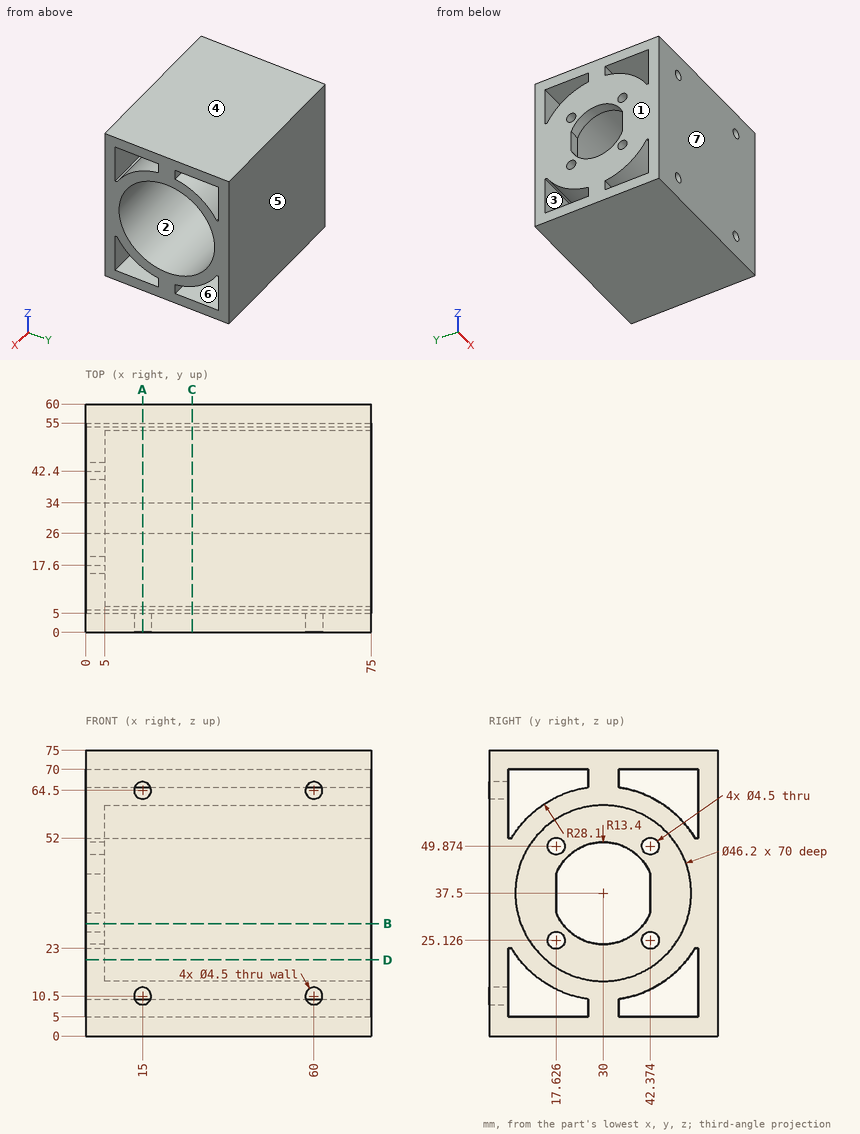
Answer from the drawing. Dimensions are ordinates in mm from the lowest x, y and z of the part. A direction names the side the tool comes from. Give positions to 0.01 mm unless a question says otherwise; leave off trailing zeros. Order: outer loops, then holes, each group sorted by start corner. A loop starts at its lowest first (then second) coordinate and runs counter-clockwise, first axis right, second up. Notation, with made-up numbers: (69, 73) - (78, 73) arc R11 cw to (78, 80) - close; hole circle Ø5 at (9.5, 60.25). An arc over 180 degrees is marked (long way). One line per item, written item: value. Start each with the question number.
1. Section C-C, the plane x = 28 is taken. Write down the section's boundary in (y, z), then the cut area to 3 significant figures.
2. Which of the six approach directions +Z, -Z, +X, -X, +Y, -Y give full straight-line access (tool end or side, diameter ignored) to the marked faces 1, 2 and 3?
3. Section A-A, the plane x = 15 is taken. Count the separate pieces of the cut face and the enclosed holes in it, then the cut area to 3 significant figures.
4. For a pull along Y with two mould halves and no side action, classify the marked faces 4, 5, 6 and 7 as released by +Y, released by -Y, zero draft, split by the parting line, or undercut.
5. Consider line 1 (X direction, y = 1.85, z = 10.5); line 2 (Y direction, x = 72.5, z = 57) (1 decimal); line 3 (Z direction, x = 69.5, y = 46.5) (1 decimal). Determine where each line is inside the solid, lowest interval first.
6. This flat-tipped pin is pushed along its axis until it touches: pin 1 Ø10 at (y, z) = (26, 34) entering from -X. Where does it stop, or does it pass through?
7. Section D-D, the plane z = 20 is taken. Write down the section's boundary in (x, y) (1 decimal).
8. Section B-B, the plane z = 29.5 is taken. Write down the section's boundary in (x, y).
Filled sheet:
1. outline: (0, 0) - (60, 0) - (60, 75) - (0, 75) - close; hole (5, 5) - (26, 5) - (26, 9.69) arc R28.1 cw to (5.93, 23) - (5, 23) - close; hole (5, 52) - (5.93, 52) arc R28.1 cw to (26, 65.31) - (26, 70) - (5, 70) - close; hole circle Ø46.2 at (30, 37.5); hole (34, 5) - (55, 5) - (55, 23) - (54.07, 23) arc R28.1 cw to (34, 9.69) - close; hole (34, 65.31) arc R28.1 cw to (54.07, 52) - (55, 52) - (55, 70) - (34, 70) - close
1. area: 2,020 mm²
2. face 1: +Z, -Z, -X, +Y, -Y
2. face 2: +X
2. face 3: +X, -X
3. separate pieces: 1
3. enclosed holes: 3
3. area: 1,980 mm²
4. face 4: zero draft
4. face 5: released by +Y
4. face 6: undercut
4. face 7: released by -Y
5. line 1: 0 to 12.75, 17.25 to 57.75, 62.25 to 75
5. line 2: 0 to 5, 9.8 to 17.6, 42.4 to 50.2, 55 to 60
5. line 3: 0 to 5, 14.8 to 21.3, 53.7 to 60.2, 70 to 75
6. pin 1: through
7. outline: (0, 0) - (75, 0) - (75, 5) - (0, 5) - close; (0, 8) - (75, 8) - (75, 14.9) - (5, 14.9) - (5, 45.1) - (75, 45.1) - (75, 52) - (0, 52) - close; (0, 55) - (75, 55) - (75, 60) - (0, 60) - close
8. outline: (0, 0) - (75, 0) - (75, 8.33) - (5, 8.33) - (5, 19.25) - (0, 19.25) - close; (0, 40.75) - (5, 40.75) - (5, 51.67) - (75, 51.67) - (75, 60) - (0, 60) - close
